Design review of the part built by this model. Coordinates are the model's own, in mm. Face numbers are marked on the shaded views. A direction names the side the tool comes from. Coordinates: 2 decimals unless noted, no trailing zeros. Write each loop counter-clockwise with the first axis right and the second up, starting at its lowest first coordinate (ties: lowest second). Pieces come first, ordered by that corner, then holes.
Q1. For L1, parallel to X at y = 4, z = 0.7 (3 decimals); L2, parallel to Y at x = -33.5, z = 2.6 (3 decimals); L3, parallel to Y at x = -34.75, z = 0.55 (3 decimals), list the stretches that pass through material, from the lowest coordinate up.
Q2. Take a section at A-A, the plane y = 6.5. Write out the cut boundary in (x, z) (3 decimals), plus the area to 3 significant figures.
Q3. Take a section at B-B, the plane x = -32. Write out the cut boundary in (y, z) (3 decimals).
Q4. Take a section at D-D, the plane x = -33.5. Write out the cut boundary in (y, z) (3 decimals), plus the area to 3 significant figures.
Q5. Take a section at C-C, the plane z = 2.1. Write out the cut boundary in (x, y) (3 decimals).
Q6. For the marked faces 1 and 2, list the 3-axis set-ups (+Z, -Z, +X, -X, +Y, -Y) from which the entire face can be reached by the end or side of a thin tool; tool diameter is ignored.
Q7. The part is to be moulded in two halves that separate along Y. For the marked faces 3, 4, 5 and 6, say which applies: released by +Y, released by -Y, zero draft, split by the parting line, or undercut.
Q8. For pin 1 Ø2 at (x, y) = (-37, -6.5) entering from -Z; pin 2 Ø1 at (x, z) = (-31.5, 2) entering from +Y, all flat-tipped, find the tip position at first contact; note any pin that passes through.
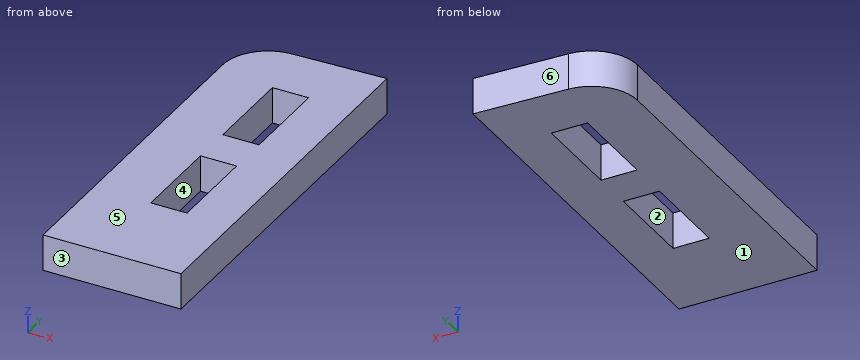
from build123d import *

# Parameters (mm, degrees)
SKETCH1_W                = 6.266
SKETCH1_H                = 19.6
SKETCH1_R                = 1.675
SKETCH1_W_2              = 52.832
SKETCH1_H_2              = 5
BOSS_EXTRUDE2_DEPTH      = 3.175
SKETCH3_W                = 30
SKETCH3_H                = 29.6
BOSS_EXTRUDE3_DEPTH      = 3.175
SKETCH4_R                = 4.85
CUT_EXTRUDE1_DEPTH       = 10
BOSS_EXTRUDE14_DEPTH     = 3.175
CUT_EXTRUDE8_DEPTH       = 10
BOSS_EXTRUDE15_DEPTH     = 3.175
BOSS_EXTRUDE16_DEPTH     = 3.175
BOSS_EXTRUDE17_DEPTH     = 3.175
FILLET5_R                = 4
SKETCH27_W               = 3.175
SKETCH27_H               = 8
CUT_EXTRUDE9_DEPTH       = 10
SKETCH28_W               = 18
SKETCH28_H               = 3.175
BOSS_EXTRUDE18_DEPTH     = 3.175
CUT_EXTRUDE10_DEPTH      = 53.993803893
CUT_EXTRUDE10_DEPTH_BACK = 53.993803893
SKETCH29_W               = 80.680500577
SKETCH29_H               = 41.601075076


with BuildPart() as part:
    # Sketch1 → Boss-Extrude2 (new body)
    # profile 1 of 4: a face of its own
    with BuildSketch(Plane.XY):
        with Locations((-23.283, 0)):
            Rectangle(SKETCH1_W, SKETCH1_H)
        with Locations((-23.95, -4.974)):
            Circle(SKETCH1_R, mode=Mode.SUBTRACT)
        with Locations((-23.95, 4.974)):
            Circle(SKETCH1_R, mode=Mode.SUBTRACT)
    # profile 2 of 4: a face of its own
    with BuildSketch(Plane.XY):
        with Locations((23.283, 0)):
            Rectangle(SKETCH1_W, SKETCH1_H)
        with Locations((23.95, -4.974)):
            Circle(SKETCH1_R, mode=Mode.SUBTRACT)
        with Locations((23.95, 4.974)):
            Circle(SKETCH1_R, mode=Mode.SUBTRACT)
    # profile 3 of 4: a face of its own
    with BuildSketch(Plane.XY):
        with Locations((0, 12.3)):
            Rectangle(SKETCH1_W_2, SKETCH1_H_2)
    # profile 4 of 4: a face of its own
    with BuildSketch(Plane.XY):
        with Locations((0, -12.3)):
            Rectangle(SKETCH1_W_2, SKETCH1_H_2)
    extrude(amount=BOSS_EXTRUDE2_DEPTH)

    # Sketch3 → Boss-Extrude3 (add)
    with BuildSketch(Plane.XY.offset(3.175)):
        with Locations((41.416, 0)):
            Rectangle(SKETCH3_W, SKETCH3_H)
    extrude(amount=-BOSS_EXTRUDE3_DEPTH)

    # Sketch4 → Cut-Extrude1 (cut)
    with BuildSketch(Plane(origin=(0, 0, 0), x_dir=(-1, 0, 0), z_dir=(0, 0, -1))):
        with Locations((-40.576, 7.77)):
            Circle(SKETCH4_R)
    extrude(amount=-CUT_EXTRUDE1_DEPTH, mode=Mode.SUBTRACT)

    # Sketch22 → Boss-Extrude14 (add)
    with BuildSketch(Plane(origin=(0, 0, 0), x_dir=(-1, 0, 0), z_dir=(0, 0, -1))):
        with BuildLine():
            ThreePointArc((-34.680262133, 14.8), (-40.576, 16.945), (-46.471737867, 14.8))
            Line((-46.471737867, 14.8), (-34.680262133, 14.8))
        make_face()
    extrude(amount=-BOSS_EXTRUDE14_DEPTH)

    # Sketch23 → Cut-Extrude8 (cut)
    with BuildSketch(Plane(origin=(0, 0, 0), x_dir=(-1, 0, 0), z_dir=(0, 0, -1))):
        with BuildLine():
            Line((-49.751, -14.8), (-49.751, 7.77))
            ThreePointArc((-49.751, 7.77), (-48.890866804, 11.648609936), (-46.471737867, 14.8))
            Line((-46.471737867, 14.8), (-56.416, 14.8))
            Line((-56.416, 14.8), (-56.416, -14.8))
            Line((-56.416, -14.8), (-49.751, -14.8))
        make_face()
    extrude(amount=-CUT_EXTRUDE8_DEPTH, mode=Mode.SUBTRACT)

    # Sketch24 → Boss-Extrude15 (add)
    with BuildSketch(Plane(origin=(0, 0, 0), x_dir=(-1, 0, 0), z_dir=(0, 0, -1))):
        Polygon((30.625, 14.8), (26.416, 14.8), (26.416, -14.8), (27.751006616, -14.8), (30.625, -14.8), align=None)
    extrude(amount=-BOSS_EXTRUDE15_DEPTH)

    # Sketch25 → Boss-Extrude16 (add)
    with BuildSketch(Plane(origin=(0, 0, 0), x_dir=(-1, 0, 0), z_dir=(0, 0, -1))):
        Polygon((30.625, 14.8), (30.625, 9.8), (33.8, 9.8), (33.8, 1.8), (30.625, 1.8), (30.625, -1.8), (33.8, -1.8), (33.8, -9.8), (30.625, -9.8), (30.625, -14.8), (31.879074074, -14.8), (38.8, -14.8), (38.8, 14.8), align=None)
    extrude(amount=-BOSS_EXTRUDE16_DEPTH)

    # Sketch26 → Boss-Extrude17 (add)
    with BuildSketch(Plane(origin=(0, 0, 0), x_dir=(-1, 0, 0), z_dir=(0, 0, -1))):
        with BuildLine():
            ThreePointArc((-40.225848077, 16.938316019), (-37.275108655, 16.330650754), (-34.680262133, 14.8))
            Line((-34.680262133, 14.8), (38.8, 14.8))
            ThreePointArc((38.8, 14.8), (-0.708684686, 16.025831975), (-40.225848077, 16.938316019))
        make_face()
    extrude(amount=-BOSS_EXTRUDE17_DEPTH)

    # Fillet5
    fillet5_edges = [part.edges().sort_by_distance(p)[0] for p in [
        (-38.8, 14.8, 1.5875),
    ]]
    fillet(fillet5_edges, radius=FILLET5_R)

    # Sketch27 → Cut-Extrude9 (cut)
    with BuildSketch(Plane(origin=(0, 0, 0), x_dir=(-1, 0, 0), z_dir=(0, 0, -1))):
        with Locations((-43.1635, -5.8)):
            Rectangle(SKETCH27_W, SKETCH27_H)
    extrude(amount=-CUT_EXTRUDE9_DEPTH, mode=Mode.SUBTRACT)

    # Sketch28 → Boss-Extrude18 (add)
    with BuildSketch(Plane(origin=(0, 0, 0), x_dir=(-1, 0, 0), z_dir=(0, 0, -1))):
        with Locations((-40.751, -16.3875)):
            Rectangle(SKETCH28_W, SKETCH28_H)
        with Locations((-5.45, -16.3875)):
            Rectangle(SKETCH28_W, SKETCH28_H)
        with Locations((29.8, -16.3875)):
            Rectangle(SKETCH28_W, SKETCH28_H)
    extrude(amount=-BOSS_EXTRUDE18_DEPTH)

    # Sketch29 → Cut-Extrude10 (cut, two sides: drawn at the far end of the back side and taken through both)
    with BuildSketch(Plane(origin=(0, 0, 0), x_dir=(-1, 0, 0), z_dir=(0, 0, -1)).offset(-CUT_EXTRUDE10_DEPTH_BACK)):
        with Locations((-13.640250288, -3.363421895)):
            Rectangle(SKETCH29_W, SKETCH29_H)
    extrude(amount=CUT_EXTRUDE10_DEPTH + CUT_EXTRUDE10_DEPTH_BACK, mode=Mode.SUBTRACT)


solid = part.part
Responses:
1. L1: x = -38.8 to -33.8, -30.625 to -26.7
1. L2: y = -17.975 to -9.8, -1.8 to 1.8, 9.8 to 14.983
1. L3: y = -17.975 to 14.94
2. outline: (-38.8, 0) - (-33.8, 0) - (-33.8, 3.175) - (-38.8, 3.175) - close; (-30.625, 0) - (-26.7, 0) - (-26.7, 3.175) - (-30.625, 3.175) - close
2. area: 28.3 mm2
3. outline: (-17.975, 0) - (-9.8, 0) - (-9.8, 3.175) - (-17.975, 3.175) - close; (-1.8, 0) - (1.8, 0) - (1.8, 3.175) - (-1.8, 3.175) - close; (9.8, 0) - (15.033, 0) - (15.033, 3.175) - (9.8, 3.175) - close
4. outline: (-17.975, 0) - (-9.8, 0) - (-9.8, 3.175) - (-17.975, 3.175) - close; (-1.8, 0) - (1.8, 0) - (1.8, 3.175) - (-1.8, 3.175) - close; (9.8, 0) - (14.983, 0) - (14.983, 3.175) - (9.8, 3.175) - close
4. area: 53.8 mm2
5. outline: (-38.8, -17.975) - (-26.7, -17.975) - (-26.7, 15.209) arc R4984.45 ccw to (-34.937, 14.934) arc R4 ccw to (-38.8, 10.936) - close; hole (-33.8, -9.8) - (-30.625, -9.8) - (-30.625, -1.8) - (-33.8, -1.8) - close; hole (-33.8, 1.8) - (-30.625, 1.8) - (-30.625, 9.8) - (-33.8, 9.8) - close
6. face 1: -Z, +X, -X, +Y, -Y
6. face 2: +Z, -Z
7. face 3: released by -Y
7. face 4: undercut
7. face 5: zero draft
7. face 6: released by +Y
8. pin 1: stops at z = 0
8. pin 2: stops at y = 15.07
